Can you work these out from the model? Positions are in its coordinate system, mm. Face numbers are marked on the shaded views. Give positions to 0.01 mm unless a question says otherwise; leave off trailing zeros. Order: outer loops, then holes, each group sorted by start corner. A loop starts at its lowest first (then second) coordinate and runs counter-clockwise, first axis right, second up. Notation, with made-up numbers: M 13,31.5 L 23,31.5 A28 cw 23,70.5 Z; hole C 79.5,15.5 d4. An arc over 180 degrees is marked long. Use a Markdown table: item, result. Add a question column.
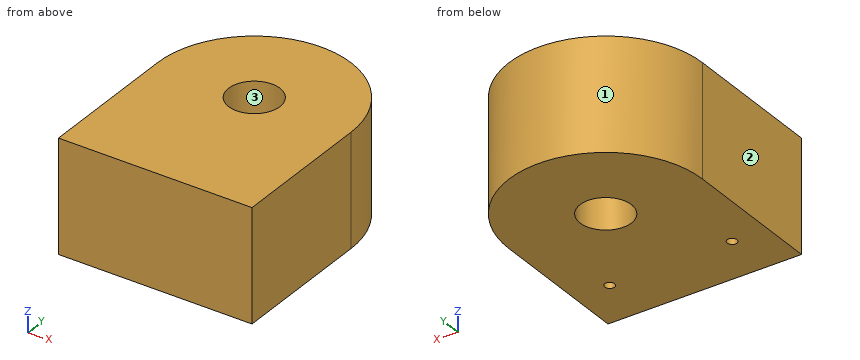
Autodesk Inventor part; units mm, degrees
ref_plane "YZ Plane" through (0, 0, 0) normal (1, 0, 0) x (0, 1, 0)
ref_plane "XZ Plane" through (0, 0, 0) normal (0, 1, 0) x (-1, 0, 0)
ref_plane "XY Plane" through (0, 0, 0) normal (0, 0, 1) x (1, 0, 0)
sketch "Sketch1" plane through (0, 0, 0) normal (0, 0, 1) x (1, 0, 0)
  line L0 (0, 73.4) -> (0, -97.4) construction
  line L1 (-68.6, 0) -> (68.6, 0) construction
  circle A0 centre (0, 0) radius 13
  arc A1 (49, 0) -> (-49, 0) centre (0, 0) ccw
  line L2 (-49, 0) -> (-49, -73)
  line L3 (-49, -73) -> (49, -73)
  line L4 (49, -73) -> (49, 0)
  dimension "d0" = 26
  dimension "d1" = 49
  dimension "d2" = 73
extrude "Extrusion1" add sketch "Sketch1" along normal mid plane 57
sketch "Sketch2" plane through (0, 0, -28.5) normal (0, 0, -1) x (-1, 0, 0)
  line L0 (-49, -73) -> (49, -73)
  point P0 (0, 0)
  point P1 (31, -48)
  point P2 (-31, -48)
  dimension "d5" = 31
  dimension "d6" = 31
  dimension "d7" = 25
hole "Hole1" at (-31, -48, -28.5) at (31, -48, -28.5) direction (0, 0, 1) diameter 4.917 depth 10 tip angle 118
properties part number "Current_transducer"
1. If we section it at D-D, the plane x = 20.5: List the corners of the cut face in (y, z) for me, then the cut area to 3 significant figures.
2. If we section it at B-B, the plane y = -9: List the corners of the cut face in (x, z) for me.
3. I need wall thicknesses on L1, parallel to X at y = -48, z = -25.25; L2, parallel to Y at x = 0, z = 15; L3, parallel to Y at x = 10, z = 1. Which ranges of each line are inside material? Lowest first, please. Write a range as [from, to].
4. If we section it at C-C, the plane z = 23: List the corners of the cut face in (x, y) for me, then the cut area to 3 significant figures.
5. If we section it at A-A, the plane x = 0: List the corners of the cut face in (y, z) for me.
6. Will these pins go through, and if not, where does the flat tip stop? pin 1 (1 mm diameter, centred on x = 18.5, z = 2.5, fed in from +Y); pin 2 (6 mm diameter, centred on y = 15, z = -7.5, fed in from +X); pin 3 (8 mm diameter, centred on x = -0.5, z = 1.5, fed in from +Y).
7. We'd pull the mould along Y, two halves only. Please class the marked faces 1, 2 and 3: +Y half, -Y half, draft (parallel to the pull), parting line (faces both ways), or undercut.
Geometry results:
| question | item | result |
|---|---|---|
| 1 | outline | M -73,-28.5 L 44.51,-28.5 L 44.51,28.5 L -73,28.5 Z |
| 1 | area | 6,700 mm^2 |
| 2 | outline | M -49,-28.5 L -9.38,-28.5 L -9.38,28.5 L -49,28.5 Z; M 9.38,-28.5 L 49,-28.5 L 49,28.5 L 9.38,28.5 Z |
| 3 | L1 | x = [-49, -33.46], [-28.54, 28.54], [33.46, 49] |
| 3 | L2 | y = [-73, -13], [13, 49] |
| 3 | L3 | y = [-73, -8.31], [8.31, 47.97] |
| 4 | outline | M -49,-73 L 49,-73 L 49,0 A49 ccw -49,0 Z; hole C 0,0 d26 |
| 4 | area | 10,400 mm^2 |
| 5 | outline | M -73,-28.5 L -13,-28.5 L -13,28.5 L -73,28.5 Z; M 13,-28.5 L 49,-28.5 L 49,28.5 L 13,28.5 Z |
| 6 | pin 1 | stops at y = 45.57 |
| 6 | pin 2 | stops at x = 47.51 |
| 6 | pin 3 | stops at y = 49 |
| 7 | face 1 | +Y half |
| 7 | face 2 | draft |
| 7 | face 3 | undercut |
